```python
from build123d import *

# Parameters (mm, degrees)
SALIENTE_EXTRUIR1_DEPTH = 8
CROQUIS2_R              = 1.75
CORTAR_EXTRUIR1_DEPTH   = 8


with BuildPart() as part:
    # Croquis1 → Saliente-Extruir1 (new body)
    with BuildSketch(Plane.XY):
        with BuildLine():
            ThreePointArc((-26.101559178, 12.607406095), (-17.021869395, -9.312904122), (4.898440822, -18.392593905))
            Line((4.898440822, -18.392593905), (53.898440822, -18.392593905))
            Line((53.898440822, -18.392593905), (53.898440822, 16.607406095))
            Line((53.898440822, 16.607406095), (-26.101559178, 16.607406095))
            Line((-26.101559178, 16.607406095), (-26.101559178, 12.607406095))
        make_face()
        with BuildLine():
            Line((-12.72677838, -7.846240232), (4.898440822, 9.77897897))
            Line((4.898440822, 9.77897897), (4.898440822, -14.392593905))
            ThreePointArc((4.898440822, -14.392593905), (-4.502398214, -12.703149518), (-12.72677838, -7.846240232))
        make_face(mode=Mode.SUBTRACT)
        Polygon((8.898440822, -14.094653751), (8.898440822, 10.220649056), (46.233665927, -14.094653751), align=None, mode=Mode.SUBTRACT)
        with BuildLine():
            Line((2.070013697, 12.607406095), (-15.555205505, -5.017813107))
            ThreePointArc((-15.555205505, -5.017813107), (-20.41211479, 3.206567059), (-22.101559178, 12.607406095))
            Line((-22.101559178, 12.607406095), (2.070013697, 12.607406095))
        make_face(mode=Mode.SUBTRACT)
        Polygon((49.898440822, 12.607406095), (49.898440822, -11.707896712), (12.563215718, 12.607406095), align=None, mode=Mode.SUBTRACT)
    extrude(amount=SALIENTE_EXTRUIR1_DEPTH)

    # Croquis2 → Cortar-Extruir1 (cut)
    with BuildSketch(Plane(origin=(0, 16.607406095, 0), x_dir=(1, 0, 0), z_dir=(0, 1, 0))):
        with Locations(Location((-17.851559178, -4, 0), (0, 0, 270))):
            Circle(CROQUIS2_R)
        with Locations(Location((45.648440822, -4, 0), (0, 0, 270))):
            Circle(CROQUIS2_R)
    extrude(amount=-CORTAR_EXTRUIR1_DEPTH, mode=Mode.SUBTRACT)


solid = part.part
```
Build history of the part. All positions in model axes, mm. A direction names the side the tool comes from. Coordinates: 2 decimals unless noted, no trailing zeros. Order: outer loops, then holes, each group sorted by start corner. A loop starts at its lowest first (then second) coordinate and runs counter-clockwise, first axis right, second up. Notation, with made-up numbers: M 87,45.5 L 120,45.5 A28 ccw 120,80.5 Z; hole C 73.5,88.25 d11. An arc over 180 degrees is marked long. One line per question, with ' | ' between items. Start each with the question number.
1. Mould opens along X. For faces 4 (the face through (28, -14.095, 4)), 5 (the face through (53.898, -1, 4)), 6 (the face through (14, 16.607, 4)) say: +X half, -X half, draft (parallel to the pull), parting line (faces both ways), or undercut.
2. Flat gauge pin, fed straight in: P1, Ø4, axis at y = 2, z = 5.5, coming from the -X side. Where does the tip first touch, or does it go through?
3. Cut at A-A (z = 1.25). Write the cut outline in (x, y).
4. Cut at B-B (y = -13). Write the cut outline in (x, z).
5. Wall check: line 1 along X through (y, z) = (15.6, 4); line 2 along X through (y, z) = (12, 7); line 3 along X through (y, z) = (7.5, 4.5). Give the ranges that are in metal, low to high. Write a range as [from, to].
6. Cut at D-D (y = 7.5). Write the cut outline in (x, z), plus the area to 3 significant figures.
7. Cut at C-C (x = -14). Write the cut outline in (y, z).
8. Tool access for faces 1 (the face through (47.384, 14.635, 3.772)), 2 (the face through (49.898, 1, 4)), 3 (the face through (13, 11, 8)): list every direction of +Z, -Z, +X, -X, +Y, -Y with a clear straight run to the whole face (end or side of a thin tool).
The answers:
1) face 4: undercut | face 5: +X half | face 6: draft
2) P1: stops at x = -24.88
3) outline: M -26.1,12.61 A31 ccw 4.9,-18.39 L 53.9,-18.39 L 53.9,16.61 L -26.1,16.61 Z; hole M -22.1,12.61 A27 ccw -15.56,-5.02 L 2.07,12.61 Z; hole M -12.73,-7.85 A27 ccw 4.9,-14.39 L 4.9,9.78 Z; hole M 8.9,-14.09 L 46.23,-14.09 L 8.9,10.22 Z; hole M 12.56,12.61 L 49.9,-11.71 L 49.9,12.61 Z
4) outline: M -12.57,0 L -3.66,0 L -3.66,8 L -12.57,8 Z; M 4.9,0 L 8.9,0 L 8.9,8 L 4.9,8 Z; M 44.55,0 L 53.9,0 L 53.9,8 L 44.55,8 Z
5) line 1: x = [-26.1, -19.6], [-16.1, 43.9], [47.4, 53.9] | line 2: x = [-26.1, -22.09], [1.46, 13.5], [49.9, 53.9] | line 3: x = [-25.68, -21.61], [-3.04, 2.62], [4.9, 8.9], [13.08, 20.41], [49.9, 53.9]
6) outline: M -25.68,0 L -21.61,0 L -21.61,8 L -25.68,8 Z; M -3.04,0 L 2.62,0 L 2.62,8 L -3.04,8 Z; M 4.9,0 L 8.9,0 L 8.9,8 L 4.9,8 Z; M 13.08,0 L 20.41,0 L 20.41,8 L 13.08,8 Z; M 49.9,0 L 53.9,0 L 53.9,8 L 49.9,8 Z | area: 200 mm2
7) outline: M -11.97,0 L -3.46,0 L -3.46,8 L -11.97,8 Z; M 12.61,0 L 16.61,0 L 16.61,8 L 12.61,8 Z
8) face 1: +Y | face 2: +Z, -Z | face 3: +Z, +X, -X, +Y, -Y
